For this review, take the finished solid that the model builds, in its own axes (mm). A direction names the side the tool comes from. Round coordinates to 2 decimals unless told otherwise and drop trailing zeros. Order: outer loops, then holes, each group sorted by start corner. A loop starts at its lowest first (then second) coordinate and runs counter-clockwise, first axis right, second up. Notation, with made-up numbers: (38.25, 83.5) -> (82.25, 83.5) arc R20 cw to (82.25, 100.5) -> close; hole circle Ø7 at (84, 31.25). An arc over 180 degrees is marked (long way). Use a Markdown table: item, result. Add a question column.
1) Consider section A-A (y = 11.52). State the section outline as (x, z) points (3 decimals).
2) Draft analysis for pull direction Z (two halves, no side actions). For faces 4 (the face through (58, 7, 0)), 5 (the face through (62, 18.657, 10)), 6 (the face through (63.36, 9.02, 9.76)), 7 (the face through (63.358, 8.39, 20.474)), state which applies: pulls with the +Z half, pulls with the -Z half, needs draft (parallel to the pull), parting line crosses it, or undercut.
3) Consider section B-B (z = 19). State the section outline as (x, y) points, plus the area to 3 significant figures.
4) Clearance check with a flat-ended pin moving along its axis: P1, Ø6.5, axis at y = 7.04, z = 19, coming from the -X side. State where the tip first meets the part, or that it passes through.
5) Consider section D-D (y = -0.5). State the section outline as (x, z) points, plus the area to 3 significant figures.
6) Consider section C-C (x = 54.25). State the section outline as (y, z) points, plus the area to 3 significant figures.
7) Wall thickness on line 1 along Y through (x, z) = (62.3, 9.5); line 2 along Z through (x, y) = (55.5, 2.25); line 3 along X through (y, z) = (-1, 6.25): over which ranges is each line inside the solid? List them lowest first. Write a range as [from, to].
8) Machinability: for faces 1 (the face through (60.985, 11.463, 3.335)), 2 (the face through (50.33, 7, 1)), 3 (the face through (61.33, 7, 14)), which of the approach directions +Z, -Z, +X, -X, +Y, -Y give a long, thin tool a straight path to every point of the face, cutting with its end or side? Answer none if there is none.
```python
from build123d import *

# Parameters (mm, degrees)
SKETCH1_W           = 15
SKETCH1_H           = 23.236534363
SKETCH1_R           = 2.58
BOSS_EXTRUDE1_DEPTH = 3
SKETCH2_W           = 4
SKETCH2_H           = 23.236534363
BOSS_EXTRUDE2_DEPTH = 20
SKETCH3_R           = 2
CUT_EXTRUDE1_DEPTH  = 4
FILLET1_R           = 2
SKETCH4_R           = 4.75
CUT_EXTRUDE2_DEPTH  = 4


with BuildPart() as part:
    # Sketch1 → Boss-Extrude1 (new body)
    with BuildSketch(Plane.XY):
        with Locations((57.83, 7.038267182)):
            Rectangle(SKETCH1_W, SKETCH1_H)
        with Locations((56.235, 11.52)):
            Circle(SKETCH1_R, mode=Mode.SUBTRACT)
    extrude(amount=BOSS_EXTRUDE1_DEPTH)

    # Sketch2 → Boss-Extrude2 (add)
    with BuildSketch(Plane.XY.offset(3)):
        with Locations((63.33, 7.038267182)):
            Rectangle(SKETCH2_W, SKETCH2_H)
    extrude(amount=BOSS_EXTRUDE2_DEPTH)

    # Sketch3 → Cut-Extrude1 (cut)
    with BuildSketch(Plane(origin=(65.33, 0, 0), x_dir=(0, 0, -1), z_dir=(1, 0, 0))):
        with Locations((-19, 7.038267182)):
            Circle(SKETCH3_R)
        with Locations((-9.5, 7.038267182)):
            Circle(SKETCH3_R)
    extrude(amount=-CUT_EXTRUDE1_DEPTH, mode=Mode.SUBTRACT)

    # Fillet1
    fillet1_edges = [part.edges().sort_by_distance(p)[0] for p in [
        (61.33, 7.038267182, 3),
    ]]
    fillet(fillet1_edges, radius=FILLET1_R)

    # Sketch4 → Cut-Extrude2 (cut)
    with BuildSketch(Plane.XY.offset(3)):
        with Locations((56.235, 11.52)):
            Circle(SKETCH4_R)
    extrude(amount=CUT_EXTRUDE2_DEPTH, mode=Mode.SUBTRACT)


solid = part.part
```
Results list:
| question | item | result |
|---|---|---|
| 1 | outline | (50.33, 0) -> (53.655, 0) -> (53.655, 3) -> (50.33, 3) -> close; (58.815, 0) -> (65.33, 0) -> (65.33, 23) -> (61.33, 23) -> (61.33, 5) arc R2 cw to (60.985, 3.877) -> (60.985, 3) -> (58.815, 3) -> close |
| 2 | face 4 | pulls with the -Z half |
| 2 | face 5 | needs draft |
| 2 | face 6 | undercut |
| 2 | face 7 | undercut |
| 3 | outline | (61.33, -4.58) -> (65.33, -4.58) -> (65.33, 5.04) -> (61.33, 5.04) -> close; (61.33, 9.04) -> (65.33, 9.04) -> (65.33, 18.66) -> (61.33, 18.66) -> close |
| 3 | area | 76.9 mm2 |
| 4 | P1 | x = 61.33 |
| 5 | outline | (50.33, 0) -> (65.33, 0) -> (65.33, 23) -> (61.33, 23) -> (61.33, 5) arc R2 cw to (59.33, 3) -> (50.33, 3) -> close |
| 5 | area | 126 mm2 |
| 6 | outline | (-4.58, 0) -> (9.87, 0) -> (9.87, 3) -> (-4.58, 3) -> close; (13.17, 0) -> (18.66, 0) -> (18.66, 3) -> (13.17, 3) -> close |
| 6 | area | 59.8 mm2 |
| 7 | line 1 | [-4.58, 5.04], [9.04, 18.66] |
| 7 | line 2 | [0, 3] |
| 7 | line 3 | [61.33, 65.33] |
| 8 | face 1 | +Z, -X |
| 8 | face 2 | +Z, -Z, -X, +Y, -Y |
| 8 | face 3 | +Z, -X, +Y, -Y |
